The listing builds one solid part. Answer for the finished solid, in the listing's coordinates (mm). A direction names the side the tool comes from. Coordinates: 2 decimals unless noted, no trailing zeros. Write each loop counter-clockwise with the first axis right and the second up, starting at its lowest first coordinate (ties: lowest second). Pieces come first, ordered by that corner, then holes.
from build123d import *

# Parameters (mm, degrees)
F2_R     = 3
F3_DEPTH = 25.4
F4_COUNT = 6


with BuildPart() as f1:
    # F0 (on Right) → F1 (revolve)
    with BuildSketch(Plane.YZ):
        Polygon((-15, 14), (-19, 14), (-19, 11), (-9.5, 11), (-9.5, 10), (-0.5, 10), (-0.5, 11), (19, 11), (19, 14), (15, 14), (15, 12), (-15, 12), align=None)
    revolve(axis=Axis((0, 0, 0), (0, 1, 0)))

    # F2 (on Top) → F3 (cut)
    with BuildSketch(Plane.XY):
        with Locations((0, -5)):
            Circle(F2_R)
    f3 = extrude(amount=-F3_DEPTH, mode=Mode.SUBTRACT)

    # F4: F3 ×6 about axis
    f4_axis = Axis((0, -19, 0), (0, 1, 0))
    for i in range(1, F4_COUNT):
        add(f3.rotate(f4_axis, i * 360 / F4_COUNT), mode=Mode.SUBTRACT)


solid = f1.part
Q1. Determine the mould class of faces 5 (the face through (10.4, -15, 6.3)), 6 (the face through (7.89, -4.1, 7.86)), 7 (the face through (-7.89, -4.1, -7.86)), 8 (the face through (-5.362, -17.028, 12.932)) for opening direction Z: released by +Z, released by -Z, zero draft, split by the parting line, or undercut.
Answers below:
face 5: zero draft
face 6: undercut
face 7: undercut
face 8: split by the parting line
Q2. Given pin 1 (1 mm diameter, centred on y = -10.5, z = -5.5, fed in from +X); pin 2 (1.5 mm diameter, centred on x = -4.5, y = 12.5, fed in from +Z); pin 3 (12 mm diameter, centred on y = 2, z = 9, fed in from +X); pin 4 (3.5 mm diameter, centred on x = 0, y = -5, fed in from +Z), each flat-ended and moving along its own axis, determine where each tip first touches the part or whether it passes through.
Answers below:
pin 1: stops at x = 10.91
pin 2: stops at z = 11.4
pin 3: stops at x = 11.62
pin 4: passes through
Q3. The part is cut by section B-B, the plane z = 0. Write down the section's boundary in (x, y), then the cut area to 3 significant figures.
Answers below:
outline: (-14, -19) - (-11, -19) - (-11, -9.5) - (-10, -9.5) - (-10, -0.5) - (-11, -0.5) - (-11, 19) - (-14, 19) - (-14, 15) - (-12, 15) - (-12, -15) - (-14, -15) - close; (10, -9.5) - (11, -9.5) - (11, -19) - (14, -19) - (14, -15) - (12, -15) - (12, 15) - (14, 15) - (14, 19) - (11, 19) - (11, -0.5) - (10, -0.5) - close
area: 126 mm2
Q4. The part is cut by section A-A, the plane x = 0. State how many separate pieces and enclosed holes the cut face has, then the cut area to 3 significant figures.
Answers below:
separate pieces: 4
enclosed holes: 0
area: 102 mm2
Q5. The part is cut by section C-C, the plane x = -3.5. Write down the section's boundary in (y, z).
Answers below:
outline: (-19, -13.56) - (-15, -13.56) - (-15, -11.48) - (15, -11.48) - (15, -13.56) - (19, -13.56) - (19, -10.43) - (-0.5, -10.43) - (-0.5, -9.37) - (-9.5, -9.37) - (-9.5, -10.43) - (-19, -10.43) - close; (-19, 10.43) - (-9.5, 10.43) - (-9.5, 9.37) - (-0.5, 9.37) - (-0.5, 10.43) - (19, 10.43) - (19, 13.56) - (15, 13.56) - (15, 11.48) - (-15, 11.48) - (-15, 13.56) - (-19, 13.56) - close
Q6. Which of the six approach directions +Z, -Z, +X, -X, +Y, -Y give full straight-line access (tool end or side, diameter ignored) to faces 1 (the face through (-10, -9.5, 2)), 2 (the face through (10.4, 15, -6.3)), 3 (the face through (-9.3, -19, 6.2)), 4 (the face through (-10.74, 9.39, -2.38))?
Answers below:
face 1: -Y
face 2: none
face 3: +Z, -Z, +X, -X, -Y
face 4: +Y
Q7. The part is cut by section D-D, the plane y = -5. Write down the section's boundary in (x, z), then the cut area to 3 significant figures.
Answers below:
outline: (-11.56, -3.21) - (-9.76, -2.17) arc R10 cw to (-9.76, 2.17) - (-11.56, 3.21) arc R12 ccw to start; (-8.56, -8.41) arc R12 ccw to (-3, -11.62) - (-3, -9.54) arc R10 cw to (-6.76, -7.37) - close; (-8.56, 8.41) - (-6.76, 7.37) arc R10 cw to (-3, 9.54) - (-3, 11.62) arc R12 ccw to start; (3, -11.62) arc R12 ccw to (8.56, -8.41) - (6.76, -7.37) arc R10 cw to (3, -9.54) - close; (3, 9.54) arc R10 cw to (6.76, 7.37) - (8.56, 8.41) arc R12 ccw to (3, 11.62) - close; (9.76, -2.17) - (11.56, -3.21) arc R12 ccw to (11.56, 3.21) - (9.76, 2.17) arc R10 cw to start
area: 65.3 mm2
Q8. Find the intervals of material crossed by probe 1 along Y at (x, z) = (0, 10.45); probe 2 along X at (y, z) = (-12.5, 0); probe 3 along X at (y, z) = (-15.75, 0), in increasing order.
Answers below:
probe 1: y = -9.5 to -8, -2 to -0.5
probe 2: x = -12 to -11, 11 to 12
probe 3: x = -14 to -11, 11 to 14
